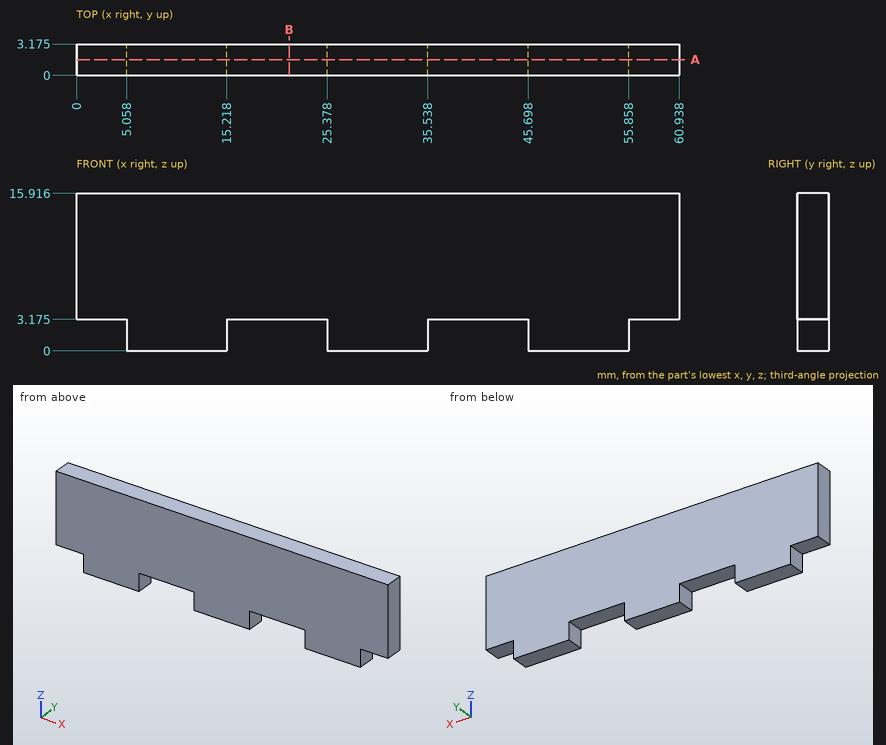
Print and shaded views of the part. All mm, measured from the part's lowest x, y and z. Coordinates: 2 decimals unless noted, no trailing zeros. Order: outer loops, then holes, each group sorted by start corner. A loop starts at its lowest first (then second) coordinate and runs counter-clockwise, first axis right, second up. Notation, with made-up numbers: (76.5, 27) - (82.5, 27) arc R20 cw to (82.5, 37) - close; hole circle Ø1 at (57, 9). An arc over 180 degrees is marked (long way). Return JSON: item names as keys, results as strings. Group by question number.
Item 1: Pin check, flat tips, straight feed: pin 1 (1 mm diameter, centred on x = 57.5, y = 1.5, fed in from -Z) (3 decimals); pin 2 (1 mm diameter, centred on y = 1, z = 1, fed in from -X). Stop position of each tip, or through.
Item 2: Cut at B-B (x = 21.5). List the corners of the cut face in (y, z) (1 decimal).
Item 3: Cut at A-A (y = 1.6). List the corners of the cut face in (x, z) (1 decimal), plus the area to 3 significant figures.
Item 4: Drill centre lines: probe 1 along X at (y, z) = (2.25, 2); probe 2 along Z at (x, y) = (17.5, 1.4) (1 decimal). Where is each one in solid material? Low to high. Write a range as from..to.
Check values:
{
 "1": {"pin 1": "stops at z = 3.175", "pin 2": "stops at x = 5.06"},
 "2": {"outline": "(0, 3.2) - (3.2, 3.2) - (3.2, 15.9) - (0, 15.9) - close"},
 "3": {"outline": "(0, 3.2) - (5.1, 3.2) - (5.1, 0) - (15.2, 0) - (15.2, 3.2) - (25.4, 3.2) - (25.4, 0) - (35.5, 0) - (35.5, 3.2) - (45.7, 3.2) - (45.7, 0) - (55.9, 0) - (55.9, 3.2) - (60.9, 3.2) - (60.9, 15.9) - (0, 15.9) - close", "area": "873 mm2"},
 "4": {"probe 1": "x = 5.06..15.22, 25.38..35.54, 45.7..55.86", "probe 2": "z = 3.2..15.9"}
}
